Can you work these out from the model? Positions are in its coordinate system, mm. A direction names the side the tool comes from. Round coordinates to 2 decimals unless told otherwise and drop trailing zeros. Loops run counter-clockwise (first coordinate to the right, second up) from the corner with the lowest first, then second, coordinate; pieces in that order, holes last.
(1) I want a section at C-C on x = -9. Write out the boundary of the cut face in (y, z) (3 decimals), plus the area to 3 significant figures.
(2) Which directions (+Z, -Z, +X, -X, +Y, -Y) give clear straight access to the entire face, cutting with the end or side of a thin tool? Please do faces 5 (the face through (27.68, 4.43, -92.07)), 6 (the face through (34, 6, -72.079)), 7 (the face through (34, 27, -89)), 8 (the face through (40.605, 4.504, -92.065)).
(3) Thinking about a two-plate mould opening in Z: for faces 1 (the face through (47.577, -0.131, -92.509)), 2 (the face through (33, 5, -58.079)), 3 (the face through (34, 3, -83)), 4 (the face through (34, 15, -91.079)), which applies, released by +Z, released by -Z, zero draft, split by the parting line, or undercut?
(4) If I drill on line 1 along Z through (x, y) = (35.5, 8.5); line 2 along Y through (x, z) = (39, -59) (3 decimals); line 3 along Y through (x, z) = (6.5, -47) (3 decimals), over which ranges is the centre line in solid material (lowest first)?
(5) Will these pins go through, and if not, where does the flat tip stop? pin 1 Ø3.5 at (x, y) = (7.5, -1) entering from -Z; pin 2 Ø6 at (x, z) = (9, -15) entering from +Y; pin 3 Ø1.8 at (y, z) = (18.5, -90) entering from -X; pin 4 Ø15.5 at (x, z) = (33, -68.5) entering from +Y.
(6) I want a section at B-B on z = -82. Write out the boundary of the cut face in (x, y) (3 decimals), plus the area to 3 significant figures.
(7) I want a section at A-A on y = 1.5. Write out the boundary of the cut face in (x, z), plus the area to 3 significant figures.
Autodesk Inventor part; units mm, degrees
ref_plane "YZ Plane" through (0, 0, 0) normal (1, 0, 0) x (0, 1, 0)
ref_plane "XZ Plane" through (0, 0, 0) normal (0, 1, 0) x (-1, 0, 0)
ref_plane "XY Plane" through (0, 0, 0) normal (0, 0, 1) x (1, 0, 0)
sketch "Sketch1" plane through (0, 0, 0) normal (0, 1, 0) x (-1, 0, 0)
  line L0 (13.8213, 11.9209) -> (-36.1787, 11.9209)
  line L1 (-38.1787, 9.9209) -> (-38.1787, -58.0791)
  line L2 (-38.1787, -58.0791) -> (13.8213, -58.0791)
  line L3 (15.8213, -56.0791) -> (15.8213, 9.9209)
  line L4 (-20.1787, -58.0791) -> (-48.1787, -58.0791)
  line L5 (-48.1787, -58.0791) -> (-48.1787, -93.0791)
  line L6 (-48.1787, -93.0791) -> (-20.1787, -93.0791)
  line L7 (-20.1787, -93.0791) -> (-20.1787, -58.0791)
  arc A0 (15.8213, 9.9209) -> (13.8213, 11.9209) centre (13.8213, 9.9209) ccw
  arc A1 (13.8213, -58.0791) -> (15.8213, -56.0791) centre (13.8213, -56.0791) ccw
  arc A2 (-36.1787, 11.9209) -> (-38.1787, 9.9209) centre (-36.1787, 9.9209) ccw
  point P0 (0, 0)
  point P1 (15.8213, 11.9209)
  point P2 (-38.1787, 11.9209)
  point P3 (15.8213, -58.0791)
  dimension "d0" = 54
  dimension "d1" = 70
  dimension "d2" = 28
  dimension "d3" = 10
  dimension "d4" = 35
  dimension "d20" = 2
extrude "Extrusion1" add sketch "Sketch1" against normal blind 3.175
sketch "Sketch2" plane through (0, 0, 0) normal (0, 1, 0) x (1, 0, 0)
  line L0 (20.1787, 93.0791) -> (20.1787, 58.0791)
  line L1 (48.1787, 58.0791) -> (48.1787, 93.0791)
  line L2 (20.1787, 93.0791) -> (48.1787, 93.0791)
  line L3 (48.1787, 93.0791) -> (48.1787, 72.0791)
  line L4 (48.1787, 72.0791) -> (20.1787, 72.0791)
  line L5 (20.1787, 72.0791) -> (20.1787, 93.0791)
  line L6 (38.1787, 58.0791) -> (48.1787, 58.0791)
  point P0 (0, 0)
  dimension "d7" = 14
extrude "Extrusion2" add sketch "Sketch2" along normal blind 3
sketch "Sketch3" plane through (0, 0, 0) normal (0, 1, 0) x (1, 0, 0)
  line L0 (48.1787, 72.0791) -> (20.1787, 72.0791)
  line L1 (48.1787, 93.0791) -> (48.1787, 58.0791)
  line L2 (20.1787, 72.0791) -> (48.1787, 72.0791)
  line L3 (48.1787, 72.0791) -> (48.1787, 58.0791)
  line L4 (48.1787, 58.0791) -> (20.1787, 58.0791)
  line L5 (20.1787, 58.0791) -> (20.1787, 72.0791)
  point P0 (0, 0)
extrude "Extrusion3" add sketch "Sketch3" along normal blind 10
ref_plane "Work Plane1" through (34.1787, -3.175, -58.0791) normal (1, 0, 0) x (0, 0, -1)
sketch "Sketch4" plane through (34.1787, -3.175, -58.0791) normal (1, 0, 0) x (0, 0, -1)
  line L0 (29, 30.175) -> (33, 30.175)
  line L1 (33, 30.175) -> (33, 6.175)
  line L2 (35, 6.175) -> (14, 6.175)
  line L3 (35, 6.175) -> (35, 35.175)
  arc A0 (35, 35.175) -> (29, 30.175) centre (35, 29.075) ccw
  point P0 (-58.0791, 3.175)
  dimension "d12" = 2
  dimension "d13" = 29
  dimension "d14" = 24
  dimension "d15" = 4
extrude "Extrusion4" add sketch "Sketch4" along normal mid plane 10
sketch "Sketch5" plane through (0, 0, 0) normal (0, 1, 0) x (1, 0, 0)
  line L0 (37.8591, -10.4638) -> (37.8591, 55.5762)
  line L1 (37.8591, 55.5762) -> (35.3191, 55.5762)
  line L2 (35.3191, 55.5762) -> (32.7791, 58.1162)
  line L3 (32.7791, 58.1162) -> (-0.2409, 58.1162)
  line L4 (-0.2409, 58.1162) -> (-2.7809, 55.5762)
  line L5 (-2.7809, 55.5762) -> (-14.2109, 55.5762)
  line L6 (-14.2109, 55.5762) -> (-15.4809, 54.3062)
  line L7 (-15.4809, 54.3062) -> (-15.4809, -10.4638)
  line L8 (-15.4809, -10.4638) -> (37.8591, -10.4638)
  spline S0 degree 3 poles (30.2391, 57.1613) (31.1145, 57.1613) (31.8242, 56.4516) (31.8242, 55.5762) (31.8242, 54.7008) (31.1145, 53.9911) (30.2391, 53.9911) (29.3637, 53.9911) (28.654, 54.7008) (28.654, 55.5762) (28.654, 56.4516) (29.3637, 57.1613) (30.2391, 57.1613) knots 0 0 0 0 1 1 1 2 2 2 3 3 3 4 4 4 4
  line L9 (30.2391, 57.1613) -> (31.1145, 57.1613) construction
  line L10 (31.1145, 57.1613) -> (31.8242, 56.4516) construction
  line L11 (31.8242, 56.4516) -> (31.8242, 55.5762) construction
  line L12 (31.8242, 55.5762) -> (31.8242, 54.7008) construction
  line L13 (31.8242, 54.7008) -> (31.1145, 53.9911) construction
  line L14 (31.1145, 53.9911) -> (30.2391, 53.9911) construction
  line L15 (30.2391, 53.9911) -> (29.3637, 53.9911) construction
  line L16 (29.3637, 53.9911) -> (28.654, 54.7008) construction
  line L17 (28.654, 54.7008) -> (28.654, 55.5762) construction
  line L18 (28.654, 55.5762) -> (28.654, 56.4516) construction
  line L19 (28.654, 56.4516) -> (29.3637, 57.1613) construction
  line L20 (29.3637, 57.1613) -> (30.2391, 57.1613) construction
  spline S1 degree 3 poles (2.2991, 57.1613) (3.1745, 57.1613) (3.8842, 56.4516) (3.8842, 55.5762) (3.8842, 54.7008) (3.1745, 53.9911) (2.2991, 53.9911) (1.4237, 53.9911) (0.714, 54.7008) (0.714, 55.5762) (0.714, 56.4516) (1.4237, 57.1613) (2.2991, 57.1613) knots 0 0 0 0 1 1 1 2 2 2 3 3 3 4 4 4 4
  line L21 (2.2991, 57.1613) -> (3.1745, 57.1613) construction
  line L22 (3.1745, 57.1613) -> (3.8842, 56.4516) construction
  line L23 (3.8842, 56.4516) -> (3.8842, 55.5762) construction
  line L24 (3.8842, 55.5762) -> (3.8842, 54.7008) construction
  line L25 (3.8842, 54.7008) -> (3.1745, 53.9911) construction
  line L26 (3.1745, 53.9911) -> (2.2991, 53.9911) construction
  line L27 (2.2991, 53.9911) -> (1.4237, 53.9911) construction
  line L28 (1.4237, 53.9911) -> (0.714, 54.7008) construction
  line L29 (0.714, 54.7008) -> (0.714, 55.5762) construction
  line L30 (0.714, 55.5762) -> (0.714, 56.4516) construction
  line L31 (0.714, 56.4516) -> (1.4237, 57.1613) construction
  line L32 (1.4237, 57.1613) -> (2.2991, 57.1613) construction
  spline S2 degree 3 poles (-12.9409, 6.3613) (-12.0655, 6.3613) (-11.3558, 5.6516) (-11.3558, 4.7762) (-11.3558, 3.9008) (-12.0655, 3.1911) (-12.9409, 3.1911) (-13.8163, 3.1911) (-14.526, 3.9008) (-14.526, 4.7762) (-14.526, 5.6516) (-13.8163, 6.3613) (-12.9409, 6.3613) knots 0 0 0 0 1 1 1 2 2 2 3 3 3 4 4 4 4
  line L33 (-12.9409, 6.3613) -> (-12.0655, 6.3613) construction
  line L34 (-12.0655, 6.3613) -> (-11.3558, 5.6516) construction
  line L35 (-11.3558, 5.6516) -> (-11.3558, 4.7762) construction
  line L36 (-11.3558, 4.7762) -> (-11.3558, 3.9008) construction
  line L37 (-11.3558, 3.9008) -> (-12.0655, 3.1911) construction
  line L38 (-12.0655, 3.1911) -> (-12.9409, 3.1911) construction
  line L39 (-12.9409, 3.1911) -> (-13.8163, 3.1911) construction
  line L40 (-13.8163, 3.1911) -> (-14.526, 3.9008) construction
  line L41 (-14.526, 3.9008) -> (-14.526, 4.7762) construction
  line L42 (-14.526, 4.7762) -> (-14.526, 5.6516) construction
  line L43 (-14.526, 5.6516) -> (-13.8163, 6.3613) construction
  line L44 (-13.8163, 6.3613) -> (-12.9409, 6.3613) construction
  spline S3 degree 3 poles (35.3191, 5.0913) (36.1945, 5.0913) (36.9042, 4.3816) (36.9042, 3.5062) (36.9042, 2.6308) (36.1945, 1.9211) (35.3191, 1.9211) (34.4437, 1.9211) (33.734, 2.6308) (33.734, 3.5062) (33.734, 4.3816) (34.4437, 5.0913) (35.3191, 5.0913) knots 0 0 0 0 1 1 1 2 2 2 3 3 3 4 4 4 4
  line L45 (35.3191, 5.0913) -> (36.1945, 5.0913) construction
  line L46 (36.1945, 5.0913) -> (36.9042, 4.3816) construction
  line L47 (36.9042, 4.3816) -> (36.9042, 3.5062) construction
  line L48 (36.9042, 3.5062) -> (36.9042, 2.6308) construction
  line L49 (36.9042, 2.6308) -> (36.1945, 1.9211) construction
  line L50 (36.1945, 1.9211) -> (35.3191, 1.9211) construction
  line L51 (35.3191, 1.9211) -> (34.4437, 1.9211) construction
  line L52 (34.4437, 1.9211) -> (33.734, 2.6308) construction
  line L53 (33.734, 2.6308) -> (33.734, 3.5062) construction
  line L54 (33.734, 3.5062) -> (33.734, 4.3816) construction
  line L55 (33.734, 4.3816) -> (34.4437, 5.0913) construction
  line L56 (34.4437, 5.0913) -> (35.3191, 5.0913) construction
  point P0 (0, 0)
extrude "Extrusion5" cut sketch "Sketch5" against normal blind 10 contours S0 | S1 | S2 | S3
fillet "Fillet1" radius 2 5 edges at (48.1787, -0.0875, -93.0791) (20.1787, -0.0875, -93.0791) (48.1787, 3.4125, -58.0791) (38.1787, -1.5875, -58.0791) (20.1787, -1.5875, -58.0791)
fillet "Fillet2" radius 5 2 edges at (39.1787, 3, -92.0791) (29.1787, 3, -92.0791)
properties part number "arduinomount"
Filled sheet:
1. outline: (-3.175, -58.079) - (0, -58.079) - (0, 11.921) - (-3.175, 11.921) - close
1. area: 222 mm2
2. face 5: -Z, -X, +Y
2. face 6: +X, -X, +Y
2. face 7: +Z, +X, -X
2. face 8: -Z, +X, +Y
3. face 1: released by -Z
3. face 2: released by +Z
3. face 3: undercut
3. face 4: undercut
4. line 1: z = -93.08 to -91.08, -72.08 to -58.08
4. line 2: y = -3.175 to 10
4. line 3: y = -3.175 to 0
5. pin 1: stops at z = -58.08
5. pin 2: stops at y = 0
5. pin 3: passes through
5. pin 4: stops at y = 10
6. outline: (20.179, -3.175) - (48.179, -3.175) - (48.179, 3) - (20.179, 3) - close
6. area: 173 mm2
7. outline: (20.18, -91.08) arc R2 ccw to (22.18, -93.08) - (46.18, -93.08) arc R2 ccw to (48.18, -91.08) - (48.18, -60.08) arc R2 ccw to (46.18, -58.08) - (20.18, -58.08) - close
7. area: 977 mm2
